Work out the finished part from the listing and answer in its coordinate system (mm). Face numbers are marked on the shaded views. A direction names the side the tool comes from. Round coordinates to 2 decimals unless told otherwise and drop trailing zeros. Order: outer loops, then holes, each group sorted by start corner. A loop starts at its lowest first (then second) coordinate and runs counter-clockwise, first axis right, second up. Notation, with made-up numbers: (-29.75, 67) - (-16.75, 67) arc R35 cw to (-16.75, 102) - close; hole circle Ø5 at (24.25, 16.25). An arc over 180 degrees is marked (long way). Put each result on its own line as item: value.
```python
from build123d import *

# Parameters (mm, degrees)
ESQUISSE1_W              = 31.25
ESQUISSE1_H              = 14.2
BOSS_EXTRU_1_DEPTH       = 1
ESQUISSE2_W              = 0.5
ESQUISSE2_H              = 0.5
BOSS_EXTRU_2_DEPTH       = 3.5
ESQUISSE3_W              = 0.5
ESQUISSE3_H              = 0.5
BOSS_EXTRU_3_DEPTH       = 0.3
ESQUISSE4_W              = 0.5
ESQUISSE4_H              = 0.5
BOSS_EXTRU_4_DEPTH       = 0.3
ESQUISSE5_R              = 2.75
BOSS_EXTRU_5_DEPTH       = 10.5
ESQUISSE6_W              = 7
ESQUISSE6_H              = 7
BOSS_EXTRU_6_DEPTH       = 4.55
ESQUISSE7_R              = 1.5
ENL_V_MAT_EXTRU_1_DEPTH  = 0.2
ESQUISSE8_W              = 1.229019946
ESQUISSE8_H              = 0.5
ESQUISSE8_W_2            = 0.5
ESQUISSE8_H_2            = 1.229019946
ENL_V_MAT_EXTRU_2_DEPTH  = 0.2
ESQUISSE9_W              = 4.73100796
ESQUISSE9_H              = 4.316007262
ESQUISSE9_W_2            = 3
ESQUISSE9_H_2            = 1
ESQUISSE9_W_3            = 0.5
ESQUISSE9_H_3            = 1.5
BOSS_EXTRU_7_DEPTH       = 0.5
ESQUISSE10_W             = 4.73100796
ESQUISSE10_H             = 4.316007262
BOSS_EXTRU_8_DEPTH       = 0.5
ESQUISSE11_R             = 1.5
ENL_V_MAT_EXTRU_3_DEPTH  = 22.5
ESQUISSE12_W             = 2.5
ESQUISSE12_H             = 7.3
BOSS_EXTRU_9_DEPTH       = 2.5
BOSS_EXTRU_10_DEPTH      = 5
BOSS_EXTRU_10_DEPTH_BACK = 4
ESQUISSE13_R             = 0.25
CONG_1_R                 = 0.25
CONG_2_R                 = 0.25
CONG_3_R                 = 0.25


with BuildPart() as part:
    # Esquisse1 → Boss.-Extru.1 (new body)
    with BuildSketch(Plane(origin=(0, 0, 0), x_dir=(1, 0, 0), z_dir=(0, 1, 0))):
        with Locations((-15.625, 7.1)):
            Rectangle(ESQUISSE1_W, ESQUISSE1_H)
    extrude(amount=BOSS_EXTRU_1_DEPTH)

    # Esquisse2 → Boss.-Extru.2 (add)
    with BuildSketch(Plane(origin=(0, 1, 0), x_dir=(1, 0, 0), z_dir=(0, 1, 0))):
        with Locations((-28.25, 12.9)):
            Rectangle(ESQUISSE2_W, ESQUISSE2_H)
        with Locations((-28.25, 1.3)):
            Rectangle(ESQUISSE2_W, ESQUISSE2_H)
    extrude(amount=BOSS_EXTRU_2_DEPTH)

    # Esquisse3 → Boss.-Extru.3 (add)
    with BuildSketch(Plane.XY.offset(-12.65)):
        with Locations((-28.25, 4.25)):
            Rectangle(ESQUISSE3_W, ESQUISSE3_H)
    extrude(amount=BOSS_EXTRU_3_DEPTH)

    # Esquisse4 → Boss.-Extru.4 (add)
    with BuildSketch(Plane(origin=(0, 0, -1.55), x_dir=(-1, 0, 0), z_dir=(0, 0, -1))):
        with Locations((28.25, 4.25)):
            Rectangle(ESQUISSE4_W, ESQUISSE4_H)
    extrude(amount=BOSS_EXTRU_4_DEPTH)

    # Esquisse5 → Boss.-Extru.5 (add)
    with BuildSketch(Plane.XY.offset(-12.35)):
        with Locations(Location((-28.25, 4.25, 0), (0, 0, 180))):
            Circle(ESQUISSE5_R)
    extrude(amount=BOSS_EXTRU_5_DEPTH)

    # Esquisse6 → Boss.-Extru.6 (add)
    with BuildSketch(Plane(origin=(0, 1, 0), x_dir=(1, 0, 0), z_dir=(0, 1, 0))):
        with Locations((-17.582259182, 10.4)):
            Rectangle(ESQUISSE6_W, ESQUISSE6_H)
    extrude(amount=BOSS_EXTRU_6_DEPTH)

    # Esquisse7 → Enlèv. mat.-Extru.1 (cut)
    with BuildSketch(Plane(origin=(0, 5.55, 0), x_dir=(1, 0, 0), z_dir=(0, 1, 0))):
        with Locations(Location((-17.582259182, 10.4, 0), (0, 0, 270))):
            Circle(ESQUISSE7_R)
    extrude(amount=-ENL_V_MAT_EXTRU_1_DEPTH, mode=Mode.SUBTRACT)

    # Esquisse8 → Enlèv. mat.-Extru.2 (cut)
    with BuildSketch(Plane(origin=(0, 5.35, 0), x_dir=(1, 0, 0), z_dir=(0, 1, 0))):
        with Locations((-18.446769155, 10.4)):
            Rectangle(ESQUISSE8_W, ESQUISSE8_H)
        with Locations((-17.582259182, 9.535490027)):
            Rectangle(ESQUISSE8_W_2, ESQUISSE8_H_2)
        with Locations((-16.717749209, 10.4)):
            Rectangle(ESQUISSE8_W, ESQUISSE8_H)
        with Locations((-17.582259182, 11.264509973)):
            Rectangle(ESQUISSE8_W_2, ESQUISSE8_H_2)
        with Locations((-17.582259182, 10.4)):
            Rectangle(ESQUISSE8_W_2, ESQUISSE8_H)
    extrude(amount=-ENL_V_MAT_EXTRU_2_DEPTH, mode=Mode.SUBTRACT)

    # Esquisse9 → Boss.-Extru.7 (add)
    with BuildSketch(Plane(origin=(0, 1, 0), x_dir=(1, 0, 0), z_dir=(0, 1, 0))):
        with Locations((-18.052754085, 3.572494065)):
            Rectangle(ESQUISSE9_W, ESQUISSE9_H)
        with Locations((-7.5, 3.5)):
            Rectangle(ESQUISSE9_W_2, ESQUISSE9_H_2)
        with Locations((-7.5, 10.7)):
            Rectangle(ESQUISSE9_W_2, ESQUISSE9_H_2)
        with Locations((-11.25, 3.75)):
            Rectangle(ESQUISSE9_W_3, ESQUISSE9_H_3)
        with Locations((-11.25, 10.45)):
            Rectangle(ESQUISSE9_W_3, ESQUISSE9_H_3)
    extrude(amount=BOSS_EXTRU_7_DEPTH)

    # Esquisse10 → Boss.-Extru.8 (add)
    with BuildSketch(Plane(origin=(0, 1.5, 0), x_dir=(1, 0, 0), z_dir=(0, 1, 0))):
        with Locations((-18.052754085, 3.572494065)):
            Rectangle(ESQUISSE10_W, ESQUISSE10_H)
    extrude(amount=BOSS_EXTRU_8_DEPTH)

    # Esquisse11 → Enlèv. mat.-Extru.3 (cut)
    with BuildSketch(Plane(origin=(0, 1, 0), x_dir=(1, 0, 0), z_dir=(0, 1, 0))):
        with Locations(Location((-7.5, 7.1, 0), (0, 0, 270))):
            Circle(ESQUISSE11_R)
    extrude(amount=-ENL_V_MAT_EXTRU_3_DEPTH, mode=Mode.SUBTRACT)

    # Esquisse12 → Boss.-Extru.9 (add)
    with BuildSketch(Plane(origin=(0, 0, 0), x_dir=(-1, 0, 0), z_dir=(0, -1, 0))):
        with Locations((1.25, 7.1)):
            Rectangle(ESQUISSE12_W, ESQUISSE12_H)
    extrude(amount=BOSS_EXTRU_9_DEPTH)

    # Esquisse13 → Boss.-Extru.10 (add, two sides: drawn at the far end of the back side and taken through both)
    with BuildSketch(Plane(origin=(0, -2.5, 0), x_dir=(-1, 0, 0), z_dir=(0, -1, 0)).offset(-BOSS_EXTRU_10_DEPTH_BACK)):
        with Locations(Location((1.25, 9.6, 0), (0, 0, 90))):
            Circle(ESQUISSE13_R)
        with Locations(Location((1.25, 7.1, 0), (0, 0, 90))):
            Circle(ESQUISSE13_R)
        with Locations(Location((1.25, 4.6, 0), (0, 0, 90))):
            Circle(ESQUISSE13_R)
    extrude(amount=BOSS_EXTRU_10_DEPTH + BOSS_EXTRU_10_DEPTH_BACK)

    # Congé1
    cong_1_edges = [part.edges().sort_by_distance(p)[0] for p in [
        (-28.5, 2.5, -1.55),
        (-28, 2.75, -1.05),
        (-28, 2.5, -1.55),
        (-28.5, 2.75, -1.05),
    ]]
    fillet(cong_1_edges, radius=CONG_1_R - 0.0001)  # a hair under: the kernel refuses the full size

    # Congé2
    cong_2_edges = [part.edges().sort_by_distance(p)[0] for p in [
        (-28.5, 4, -1.57505),
        (-28, 4, -1.57505),
        (-28.426805985, 4.5, -1.123194015),
        (-28.073194015, 4.5, -1.123194015),
        (-28.5, 4.5, -1.57495),
        (-28, 4.5, -1.57495),
    ]]
    fillet(cong_2_edges, radius=CONG_2_R - 0.0001)  # a hair under: the kernel refuses the full size

    # Congé3
    cong_3_edges = [part.edges().sort_by_distance(p)[0] for p in [
        (-28, 4, -12.5),
        (-28, 2.5, -12.65),
        (-28, 2.75, -13.15),
        (-28, 4.5, -12.75),
        (-28.5, 2.5, -12.65),
        (-28.5, 4, -12.5),
        (-28.5, 4.5, -12.75),
        (-28.5, 2.75, -13.15),
    ]]
    fillet(cong_3_edges, radius=CONG_3_R - 0.0001)  # a hair under: the kernel refuses the full size


solid = part.part
```
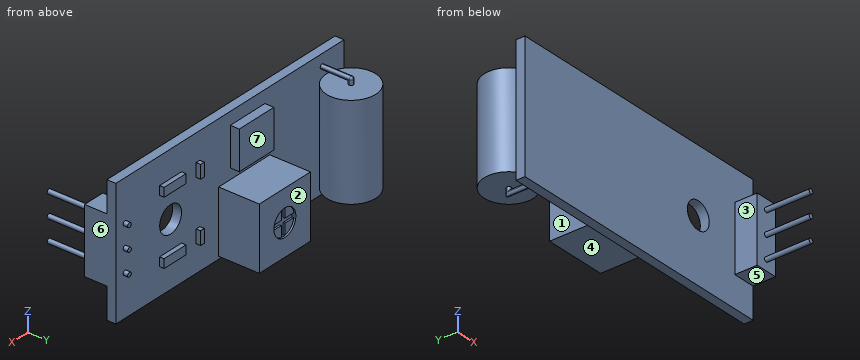
1) A cutting plane is placed at D-D on y = -2. Write down the section's boundary in (x, z).
Findings below:
outline: (-2.5, -10.75) - (0, -10.75) - (0, -3.45) - (-2.5, -3.45) - close
2) A cutting plane is placed at C-C on z = -11.5. Write down the section's boundary in (x, y), then the cut area to 3 significant figures.
Findings below:
outline: (-31.25, 0) - (0, 0) - (0, 1) - (-14.08, 1) - (-14.08, 5.55) - (-16.56, 5.55) - (-16.56, 5.35) - (-17.33, 5.35) - (-17.33, 5.15) - (-17.83, 5.15) - (-17.83, 5.35) - (-18.6, 5.35) - (-18.6, 5.55) - (-21.08, 5.55) - (-21.08, 1) - (-31.25, 1) - close; circle Ø5.5 at (-28.25, 4.25)
area: 86.4 mm2
3) Straight lines are drawn through the part: L1, parallel to X at y = 0.8, z = -7.1; L2, parallel to X at y = 5.45, z = -10.4; L3, parallel to Y at x = -6, z = -1.5. For each, find the intervals that lie inside material, in ascending order. Write a range as from..to.
Findings below:
L1: x = -31.25..-9, -6..0
L2: x = -30.72..-25.78, -21.08..-19.08, -16.08..-14.08
L3: y = 0..1
4) Given pin 1 Ø1.5 at (x, z) = (-13, -11) entering from -Y; pin 2 Ø1.6 at (x, y) = (-27.5, 3) entering from -Z; pin 3 Ø3 at (y, z) = (-3.5, -10.5) entering from -X; pin 4 Ø2 at (x, y) = (-26.5, -1.5) entering from +Z, each flat-ended and moving along its own axis, determine where each tip first touches the part or whether it passes through.
Findings below:
pin 1: stops at y = 0
pin 2: stops at z = -13.15
pin 3: stops at x = -2.5
pin 4: passes through
5) A cutting plane is placed at B-B on z = -8. Write down the section's boundary in (x, y).
Findings below:
outline: (-31.25, 0) - (-8.7, 0) - (-8.7, 1) - (-14.08, 1) - (-14.08, 5.55) - (-21.08, 5.55) - (-21.08, 1) - (-31.25, 1) - close; circle Ø5.5 at (-28.25, 4.25); (-6.3, 0) - (-2.5, 0) - (-2.5, -2.5) - (0, -2.5) - (0, 1) - (-6.3, 1) - close
6) A cutting plane is placed at A-A on x = -7.5. Write down the section's boundary in (y, z).
Findings below:
outline: (0, -14.2) - (1, -14.2) - (1, -11.2) - (1.5, -11.2) - (1.5, -10.2) - (1, -10.2) - (1, -8.6) - (0, -8.6) - close; (0, -5.6) - (1, -5.6) - (1, -4) - (1.5, -4) - (1.5, -3) - (1, -3) - (1, 0) - (0, 0) - close
7) For the marked faces 4, 5, 6 and 7, determine the directions among +Z, -Z, +X, -X, +Y, -Y from which every point of the face is accessible in a straight line to the end or side of a thin tool.
Findings below:
face 4: -Z, +X, -X, +Y
face 5: -Z, +X, -X, -Y
face 6: +Z, -Z, +X, +Y, -Y
face 7: +Z, +X, +Y
8) For a pull along X with two mould halves and no side action, classify the marked faces 1, 2 and 3 as pulls with the +X half, pulls with the -X half, needs draft (parallel to the pull), parting line crosses it, or undercut.
Findings below:
face 1: undercut
face 2: needs draft
face 3: pulls with the -X half
